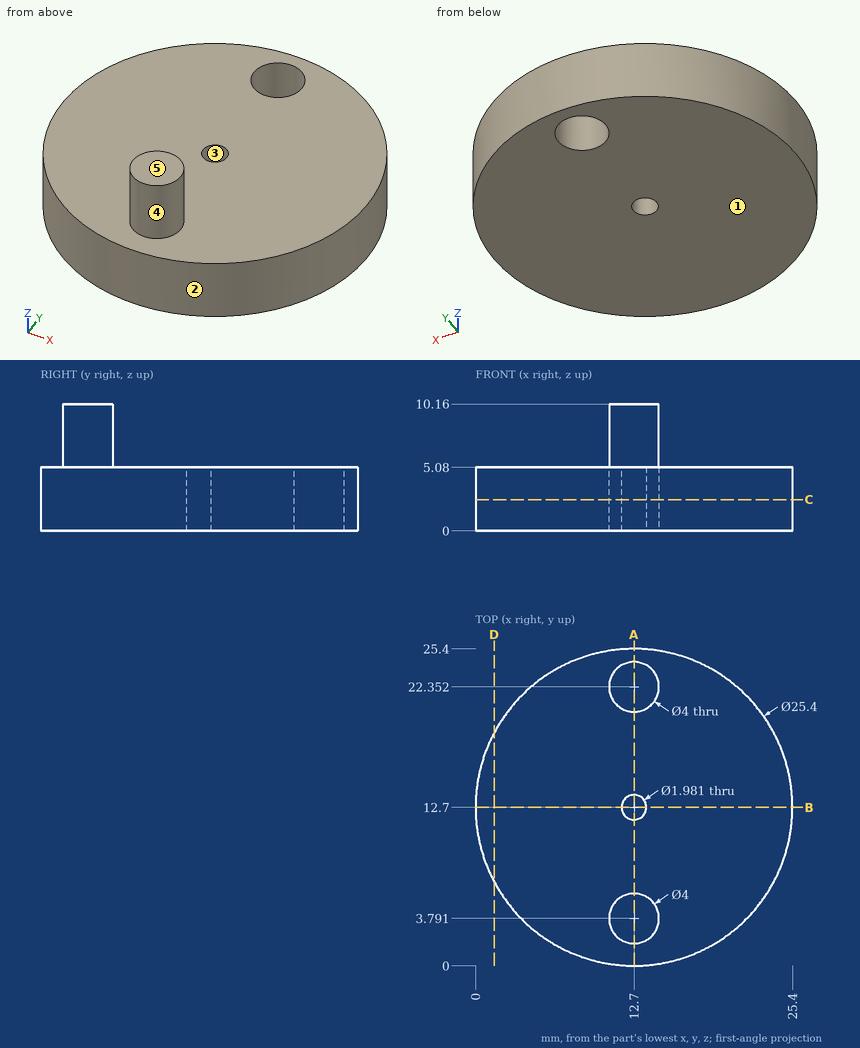
Geometry check sheet. Reference: drawing and pictorial views, mm from the part's lowest x, y, z. A direction names the side the tool comes from. Give positions to 0.01 mm unless a question says otherwise; leave off trailing zeros. Order: outer loops, then holes, each group sorted by start corner. A loop starts at its lowest first (then second) coordinate and runs counter-clockwise, first axis right, second up. Notation, with made-up numbers: M 32.5,20.5 L 73.5,20.5 A11 cw 73.5,31.5 Z; hole C 49,14 d5. An arc over 180 degrees is marked long. Return JSON: item names as keys, results as strings. Group by question number.
1) Section check A-A on x = 12.7. Record the cut outline in (y, z), and give its area (3 significant figures).
2) Go/stop test with flat-tipped pins: pin 1 Ø4 at (x, z) = (14, 7) entering from +Y; pin 2 Ø5 at (y, z) = (16.5, 6) entering from -X; pin 3 Ø5 at (x, z) = (9, 5) entering from -Y. Record where each tip stops, or that it passes through.
3) Section check C-C on z = 2.5. Record the cut outline in (x, y).
4) Scan lines: line 1 (Y direction, x = 12.7, z = 2.9); line 2 (Z direction, x = 7.5, y = 7.25); line 3 (X direction, y = 22.5, z = 2.25) (1 decimal). Record each from-to range of solid material in increasing order.
5) Mould release check, pull along Y, two halves, no side actions. Record for the marked faces 1, 2 and 3: pulls with the +Y half, pulls with the -Y half, needs draft (parallel to the pull), parting line crosses it, or undercut.
6) Section check B-B on y = 12.7. Record the cut outline in (x, z), and give its area (3 significant figures).
7) Access from +Z, -Z, +X, -X, +Y, -Y to the whole of each face (thin tool, end or side, straight path). Record for the marked faces 4 and 5.
8) Section check D-D on x = 1.5. Record the cut outline in (y, z), and give its area (3 significant figures).
Answer block:
{
 "1": {"outline": "M 0,0 L 11.71,0 L 11.71,5.08 L 5.79,5.08 L 5.79,10.16 L 1.79,10.16 L 1.79,5.08 L 0,5.08 Z; M 13.69,0 L 20.35,0 L 20.35,5.08 L 13.69,5.08 Z; M 24.35,0 L 25.4,0 L 25.4,5.08 L 24.35,5.08 Z", "area": "119 mm^2"},
 "2": {"pin 1": "stops at y = 25.38", "pin 2": "stops at x = 0.09", "pin 3": "stops at y = 0.06"},
 "3": {"outline": "C 12.7,12.7 d25.4; hole C 12.7,22.35 d4; hole C 12.7,12.7 d1.98"},
 "4": {"line 1": "y = 0 to 11.71, 13.69 to 20.35, 24.35 to 25.4", "line 2": "z = 0 to 5.08", "line 3": "x = 4.6 to 10.7, 14.7 to 20.8"},
 "5": {"face 1": "needs draft", "face 2": "parting line crosses it", "face 3": "undercut"},
 "6": {"outline": "M 0,0 L 11.71,0 L 11.71,5.08 L 0,5.08 Z; M 13.69,0 L 25.4,0 L 25.4,5.08 L 13.69,5.08 Z", "area": "119 mm^2"},
 "7": {"face 4": "+Z", "face 5": "+Z, +X, -X, +Y, -Y"},
 "8": {"outline": "M 6.71,0 L 18.69,0 L 18.69,5.08 L 6.71,5.08 Z", "area": "60.8 mm^2"}
}
